from build123d import *

# Parameters (mm, degrees)
SKETCH3_R                = 3.81
DOWELSUPPORT_DEPTH       = 1.27
SKETCH5_W                = 6.35
SKETCH5_H                = 31.75
SLIDERDOWELSUPPORT_DEPTH = 1.27
STRINGDOWELSUPPORT_DEPTH = 1.27
SKETCH9_W                = 6.35
SKETCH9_H                = 3
TABSUPPORT_DEPTH         = 1.27
INTERSUPPORT_DEPTH       = 1.27
DOWELHOLES_DEPTH         = 36.066951521
DOWELHOLES_DEPTH_BACK    = 36.066951521
SKETCH11_R               = 1.690500048
SKETCH14_W               = 6.35
SKETCH14_H               = 3
TABBASE_DEPTH            = 1.27
SKETCH15_W               = 6.35
SKETCH15_H               = 3
TABDRAFT_DEPTH           = 1.73
TABDRAFT_DRAFT           = 5
TABDRAFT_PROFILE_2_DEPTH = 1.73
TABDRAFT_PROFILE_2_DRAFT = 5


with BuildPart() as part:
    # Sketch3 → DowelSupport (new, symmetric)
    with BuildSketch(Plane(origin=(0, 0, 0), x_dir=(0, 0, -1), z_dir=(1, 0, 0))):
        with Locations((-3.175, 26.19375)):
            Circle(SKETCH3_R)
    extrude(amount=DOWELSUPPORT_DEPTH, both=True)



with BuildPart() as body_2:
    # Sketch5 → SliderDowelSupport (new, symmetric)
    with BuildSketch(Plane(origin=(0, 0, 0), x_dir=(0, 0, -1), z_dir=(1, 0, 0))):
        Rectangle(SKETCH5_W, SKETCH5_H)
    extrude(amount=SLIDERDOWELSUPPORT_DEPTH, both=True)


with BuildPart() as body_3:
    # Sketch8 → StringDowelSupport (new, symmetric)
    with BuildSketch(Plane(origin=(0, 0, 0), x_dir=(0, 0, -1), z_dir=(1, 0, 0))):
        with BuildLine():
            Line((4.6355, 31.242), (8.0645, 31.242))
            ThreePointArc((8.0645, 31.242), (10.6045, 28.702), (8.0645, 26.162))
            Line((8.0645, 26.162), (4.6355, 26.162))
            ThreePointArc((4.6355, 26.162), (2.0955, 28.702), (4.6355, 31.242))
        make_face()
    extrude(amount=STRINGDOWELSUPPORT_DEPTH, both=True)


with BuildPart() as part_1:
    add(part.part)

    add(body_3.part)  # TabSupport merges body 3
    # Sketch9 → TabSupport (add, symmetric)
    with BuildSketch(Plane(origin=(0, 0, 0), x_dir=(0, 0, -1), z_dir=(1, 0, 0))):
        with Locations((0, 27.94)):
            Rectangle(SKETCH9_W, SKETCH9_H)
        with Locations((12.7, 27.94)):
            Rectangle(SKETCH9_W, SKETCH9_H)
    extrude(amount=TABSUPPORT_DEPTH, both=True)


    add(body_2.part)  # InterSupport merges body 2
    # Sketch10 → InterSupport (add, symmetric)
    with BuildSketch(Plane(origin=(0, 0, 0), x_dir=(0, 0, -1), z_dir=(1, 0, 0))):
        Polygon((-3.175, 15.875), (-5.636846154, 25.568519231), (-3.951626852, 28.612107032), (3.858873148, 31.120357032), (8.657140431, 31.171894192), (15.875, 29.44), (15.875, 26.44), (3.175, 9.525), (3.175, 15.875), align=None)
    extrude(amount=INTERSUPPORT_DEPTH, both=True)

    # Sketch11 → DowelHoles (cut, two sides: drawn at the far end of the back side and taken through both)
    with BuildSketch(Plane(origin=(0, 0, 0), x_dir=(0, 0, -1), z_dir=(1, 0, 0)).offset(-DOWELHOLES_DEPTH_BACK)):
        with Locations((-3.175, 26.19375)):
            Circle(SKETCH11_R)
        with BuildLine():
            Line((6.144521674, 27.94), (6.555478326, 27.94))
            ThreePointArc((6.555478326, 27.94), (9.755000048, 28.702), (6.555478326, 29.464))
            Line((6.555478326, 29.464), (6.144521674, 29.464))
            ThreePointArc((6.144521674, 29.464), (2.944999952, 28.702), (6.144521674, 27.94))
        make_face()
    extrude(amount=DOWELHOLES_DEPTH + DOWELHOLES_DEPTH_BACK, mode=Mode.SUBTRACT)

    # Sketch14 → TabBase (add)
    with BuildSketch(Plane.ZY.offset(1.27)):
        with Locations((-12.7, 27.94)):
            Rectangle(SKETCH14_W, SKETCH14_H)
        with Locations((0, 27.94)):
            Rectangle(SKETCH14_W, SKETCH14_H)
    extrude(amount=TABBASE_DEPTH)


with BuildPart() as tabdraft_tool:
    # Sketch15 → TabDraft (with draft: the straight prism first)
    with BuildSketch(Plane.ZY.offset(2.54)):
        with Locations((0, 27.94)):
            Rectangle(SKETCH15_W, SKETCH15_H)
    extrude(amount=TABDRAFT_DEPTH)
    # TabDraft: the draft: its side faces are tilted about the plane it starts from
    tabdraft_sides = [tabdraft_tool.faces().sort_by_distance(p)[0] for p in [
        (-3.405, 27.94, -3.175),
        (-3.405, 26.44, 0),
        (-3.405, 27.94, 3.175),
        (-3.405, 29.44, 0),
    ]]
    draft(tabdraft_sides, Plane.ZY.offset(2.54), TABDRAFT_DRAFT)


with BuildPart() as part_2:
    add(part_1.part)

    # TabDraft: add tabdraft_tool
    add(tabdraft_tool.part)


with BuildPart() as tabdraft_profile_2_tool:
    # Sketch15 → TabDraft profile 2 (with draft: the straight prism first)
    with BuildSketch(Plane.ZY.offset(2.54)):
        with Locations((-12.7, 27.94)):
            Rectangle(SKETCH15_W, SKETCH15_H)
    extrude(amount=TABDRAFT_PROFILE_2_DEPTH)
    # TabDraft profile 2: the draft: its side faces are tilted about the plane it starts from
    tabdraft_profile_2_sides = [tabdraft_profile_2_tool.faces().sort_by_distance(p)[0] for p in [
        (-3.405, 27.94, -15.875),
        (-3.405, 26.44, -12.7),
        (-3.405, 27.94, -9.525),
        (-3.405, 29.44, -12.7),
    ]]
    draft(tabdraft_profile_2_sides, Plane.ZY.offset(2.54), TABDRAFT_PROFILE_2_DRAFT)


with BuildPart() as part_3:
    add(part_2.part)

    # TabDraft profile 2: add tabdraft_profile_2_tool
    add(tabdraft_profile_2_tool.part)

    # Mirror1: part across plane


with BuildPart() as part_4:
    add(part_3.part)
    add(part_3.part.mirror(Plane.ZX))


solid = part_4.part
CAD build for the part. Positions are in the model's coordinates, mm. A direction names the side the tool comes from. Round coordinates to 2 decimals unless told otherwise and drop trailing zeros. Write each loop counter-clockwise with the first axis right and the second up, starting at its lowest first coordinate (ties: lowest second). Pieces come first, ordered by that corner, then holes. Notation, with made-up numbers: M 13.25,3 L 61.25,3 A17 ccw 61.25,36 Z; hole C 20.5,24.5 d1. An arc over 180 degrees is marked long. Use a Markdown table: item, result. Add a question column.
1. Slice it at A-A on z = -7.5. Give the cut face in (x, y).
2. Slice it at B-B on x = -0.55. Give the number of separate pieces and of enclosed holes in the cut face, then the cut area to 3 significant figures.
3. Slice it at C-C on z = 0.5. Give the cut face in (x, y), then the cut area to 3 significant figures.
4. Pull direction Z, two halves, no side cores. Call faces 1 (the face through (-2, -28, 3.175)), 2 (the face through (0.02, 28.11, 6.47)), 3 (the face through (-2, 29.44, 0)), 4 (the face through (-1, -28, -15.875)): released by +Z, released by -Z, zero draft, split by the parting line, or undercut.
5. Drill centre lines: probe 1 along Z at (x, y) = (-2.3, 26.5) (3 decimals); probe 2 along Y at (x, z) = (-1.1, -7.5); probe 3 along X at (y, z) = (-23, -1.5). Where is each one in solid material? Low to high.
6. 3-axis set-ups, long thin cutter, end or side, ignore diameter. For faces 5 (the face through (0.018, 19.297, 4.044)), 6 (the face through (0.018, 18.101, -9.614)), 7 (the face through (-1.27, -27, 3)), 8 (the face through (-3.393, 26.515, -0.044)): which of +Z, -Z, +X, -X, +Y, -Y reach the whole face in a straight line?
7. Flat gauge pins, fed straight in: P1, Ø10, axis at y = 12.5, z = 3, coming from the -X side; P2, Ø1.3, axis at x = 0, y = -1.5, coming from the -Z side (3 decimals); P3, Ø3, axis at x = -0.5, y = 5.5, coming from the +Z side (3 decimals). Where does each tip first touch, or does it go through?
8. Slice it at D-D on y = 1. Give the cut face in (x, z) (3 decimals).
Reply:
| question | item | result |
|---|---|---|
| 1 | outline | M -1.27,-31.24 L 1.27,-31.24 L 1.27,-30.3 L -1.27,-30.3 Z; M -1.27,-27.11 L 1.27,-27.11 L 1.27,-15.29 L -1.27,-15.29 Z; M -1.27,15.29 L 1.27,15.29 L 1.27,27.11 L -1.27,27.11 Z; M -1.27,30.3 L 1.27,30.3 L 1.27,31.24 L -1.27,31.24 Z |
| 2 | separate pieces | 1 |
| 2 | enclosed holes | 4 |
| 2 | area | 707 mm^2 |
| 3 | outline | M -4.27,-29.29 L -2.54,-29.44 L -1.27,-29.44 L -1.27,-29.72 L 1.27,-29.72 L 1.27,29.72 L -1.27,29.72 L -1.27,29.44 L -2.54,29.44 L -4.27,29.29 L -4.27,26.59 L -2.54,26.44 L -1.27,26.44 L -1.27,-26.44 L -2.54,-26.44 L -4.27,-26.59 Z |
| 3 | area | 168 mm^2 |
| 4 | face 1 | released by +Z |
| 4 | face 2 | undercut |
| 4 | face 3 | zero draft |
| 4 | face 4 | released by -Z |
| 5 | probe 1 | z = -15.875 to -9.525, -3.175 to 3.175 |
| 5 | probe 2 | y = -31.24 to -30.3, -27.11 to -15.29, 15.29 to 27.11, 30.3 to 31.24 |
| 5 | probe 3 | x = -1.27 to 1.27 |
| 6 | face 5 | +Z, +X, -X |
| 6 | face 6 | -Z, +X, -X |
| 6 | face 7 | +X |
| 6 | face 8 | +Z, -Z, -X |
| 7 | P1 | stops at x = -1.27 |
| 7 | P2 | stops at z = -3.175 |
| 7 | P3 | stops at z = 3.175 |
| 8 | outline | M -1.27,-3.175 L 1.27,-3.175 L 1.27,3.175 L -1.27,3.175 Z |
